```python
from build123d import *

# Parameters (mm, degrees)
SKETCH_2_R          = 19
SKETCH_2_R_2        = 2.75
EXTRUDE_1_DEPTH     = 14
SKETCH_3_R          = 21.125
CUT_EXTRUDE_1_DEPTH = 12.15
FILLET_1_R          = 8
SKETCH_5_R          = 0.9
CUT_EXTRUDE_3_DEPTH = 61.017185039
SKETCH_6_R          = 21.125
SKETCH_6_R_2        = 2.75
EXTRUDE_2_DEPTH     = 14
CUT_EXTRUDE_4_DEPTH = 13
SKETCH_8_R          = 2
CUT_EXTRUDE_5_DEPTH = 2
FILLET_2_R          = 1
CUT_EXTRUDE_6_REACH = 77.034
CHAMFER_1_SIZE      = 1


with BuildPart() as part:
    # Эскиз2 → Бобышка-Вытянуть1 (new body)
    with BuildSketch(Plane.XY):
        with BuildLine():
            ThreePointArc((26, 26.25), (0, 52.25), (-26, 26.25))
            Line((-26, 26.25), (-26, -20))
            Line((-26, -20), (26, -20))
            Line((26, -20), (26, 26.25))
        make_face()
        with Locations((0, 26.25)):
            Circle(SKETCH_2_R, mode=Mode.SUBTRACT)
        with Locations((12, -10)):
            Circle(SKETCH_2_R_2, mode=Mode.SUBTRACT)
        with Locations((-12, -10)):
            Circle(SKETCH_2_R_2, mode=Mode.SUBTRACT)
    extrude(amount=EXTRUDE_1_DEPTH)

    # Эскиз3 → Вырез-Вытянуть1 (cut)
    with BuildSketch(Plane.XY.offset(14)):
        with Locations((0, 26.25)):
            Circle(SKETCH_3_R)
    extrude(amount=-CUT_EXTRUDE_1_DEPTH, mode=Mode.SUBTRACT)

    # Скругление1
    fillet_1_edges = [part.edges().sort_by_distance(p)[0] for p in [
        (26, -20, 7),
        (-26, -20, 7),
    ]]
    fillet(fillet_1_edges, radius=FILLET_1_R)

    # Эскиз5 → Вырез-Вытянуть3 (cut, through all)
    with BuildSketch(Plane.XY.offset(14)):
        with Locations((0, 49.75)):
            Circle(SKETCH_5_R)
        with Locations((-23.5, 26.25)):
            Circle(SKETCH_5_R)
        with Locations((23.5, 26.25)):
            Circle(SKETCH_5_R)
        with Locations((-22, -10)):
            Circle(SKETCH_5_R)
        with Locations(Location((22, -10, 0), (0, 0, 180))):
            Circle(SKETCH_5_R)
    extrude(amount=-CUT_EXTRUDE_3_DEPTH, mode=Mode.SUBTRACT)

    # Эскиз6 → Бобышка-Вытянуть2 (add, through all)
    with BuildSketch(Plane.XY.offset(14)):
        with Locations((0, 26.25)):
            Circle(SKETCH_6_R)
        with Locations((-12, -10)):
            Circle(SKETCH_6_R_2)
        with Locations((12, -10)):
            Circle(SKETCH_6_R_2)
    extrude(amount=-EXTRUDE_2_DEPTH)

    # Эскиз7 → Вырез-Вытянуть4 (cut)
    with BuildSketch(Plane(origin=(0, 0, 0), x_dir=(-1, 0, 0), z_dir=(0, 0, -1))):
        with BuildLine():
            Line((-23.5, 21.75), (-24, 21.75))
            Line((-24, 21.75), (-24, -5.5))
            Line((-24, -5.5), (-22, -5.5))
            ThreePointArc((-22, -5.5), (-18.818019485, -6.818019485), (-17.5, -10))
            Line((-17.5, -10), (-17.5, -18))
            Line((-17.5, -18), (17.5, -18))
            Line((17.5, -18), (17.5, -10))
            ThreePointArc((17.5, -10), (18.818019485, -6.818019485), (22, -5.5))
            Line((22, -5.5), (24, -5.5))
            Line((24, -5.5), (24, 21.75))
            Line((24, 21.75), (23.5, 21.75))
            ThreePointArc((23.5, 21.75), (20.318019485, 23.068019485), (19, 26.25))
            ThreePointArc((19, 26.25), (0, 45.25), (-19, 26.25))
            ThreePointArc((-19, 26.25), (-20.318019485, 23.068019485), (-23.5, 21.75))
        make_face()
    extrude(amount=-CUT_EXTRUDE_4_DEPTH, mode=Mode.SUBTRACT)

    # Эскиз8 → Вырез-Вытянуть5 (cut)
    with BuildSketch(Plane.XY.offset(14)):
        with Locations((-22, -10)):
            Circle(SKETCH_8_R)
        with Locations((22, -10)):
            Circle(SKETCH_8_R)
        with BuildLine():
            Line((2, 49.75), (2, 52.25))
            Line((2, 52.25), (-2, 52.25))
            Line((-2, 52.25), (-2, 49.75))
            ThreePointArc((-2, 49.75), (0, 47.75), (2, 49.75))
        make_face()
        with BuildLine():
            Line((26, 28.25), (23.5, 28.25))
            ThreePointArc((23.5, 28.25), (21.5, 26.25), (23.5, 24.25))
            Line((23.5, 24.25), (26, 24.25))
            Line((26, 24.25), (26, 28.25))
        make_face()
        with BuildLine():
            Line((-26, 24.25), (-23.5, 24.25))
            ThreePointArc((-23.5, 24.25), (-21.5, 26.25), (-23.5, 28.25))
            Line((-23.5, 28.25), (-26, 28.25))
            Line((-26, 28.25), (-26, 24.25))
        make_face()
    extrude(amount=-CUT_EXTRUDE_5_DEPTH, mode=Mode.SUBTRACT)

    # Скругление2
    fillet_2_edges = [part.edges().sort_by_distance(p)[0] for p in [
        (24, -5.5, 6.5),
        (17.5, -18, 6.5),
        (-17.5, -18, 6.5),
        (-24, -5.5, 6.5),
        (-24, 21.75, 6.5),
        (24, 21.75, 6.5),
        (26, 24.25, 13),
        (25.922962794, 28.25, 13),
        (2, 52.172962794, 13),
        (-2, 52.172962794, 13),
        (-26, 24.25, 13),
        (-25.922962794, 28.25, 13),
    ]]
    fillet(fillet_2_edges, radius=FILLET_2_R)

    # Эскиз9 → Вырез-Вытянуть6 (cut, up to next)
    with BuildSketch(Plane.ZY.offset(26), mode=Mode.PRIVATE) as cut_extrude_6_sk1:
        with BuildLine():
            Line((-7.5, 10.375), (4.5, 10.375))
            ThreePointArc((4.5, 10.375), (6.621320344, 9.496320344), (7.5, 7.375))
            Line((7.5, 7.375), (7.5, 6.875))
            ThreePointArc((7.5, 6.875), (6.621320344, 4.753679656), (4.5, 3.875))
            Line((4.5, 3.875), (-7.5, 3.875))
            Line((-7.5, 3.875), (-7.5, 10.375))
        make_face()
    cut_extrude_6_tool1 = extrude(cut_extrude_6_sk1.sketch, amount=-CUT_EXTRUDE_6_REACH, mode=Mode.PRIVATE) & part.part
    add(cut_extrude_6_tool1.solids().sort_by_distance((-26, 7.125, -0.281755))[0], mode=Mode.SUBTRACT)

    # Фаска1
    chamfer_1_edges = [part.edges().sort_by_distance(p)[0] for p in [
        (2, 50.409673646, 14),
        (0, 47.75, 14),
        (21.5, 26.25, 14),
        (24.25, 24.25, 14),
        (-24.159673646, 28.25, 14),
        (-21.5, 26.25, 14),
        (22.5, -5.5, 13),
        (24, 8.136387212, 13),
        (0, -18, 13),
        (-17.5, -13.5, 13),
        (-24, 8.136387212, 13),
        (-20.176529744, 23.216100619, 13),
        (23.738548946, 21.446974287, 13),
        (-23.738548945, 21.446974288, 13),
        (-23.707106781, -5.207106781, 13),
        (-17.207106781, -17.707106781, 13),
        (17.207106781, -17.707106781, 13),
        (23.707106781, -5.207106781, 13),
        (26, 5.625, 14),
        (-2, 50.409673646, 14),
        (-18.384776311, 44.634776311, 14),
        (-24.25, 24.25, 14),
        (-26, 5.625, 14),
        (24.159673646, 28.25, 14),
        (18.384776311, 44.634776311, 14),
        (-25.567678769, 28.586675042, 14),
        (-25.707106781, 23.957106781, 14),
        (-2.336675042, 51.817678769, 14),
        (2.336675042, 51.817678769, 14),
        (25.567678769, 28.586675042, 14),
        (25.707106781, 23.957106781, 14),
        (0, -20, 14),
        (23.656854249, -17.656854249, 14),
        (-23.656854249, -17.656854249, 14),
        (20.176529744, 23.216100619, 13),
        (0, 45.25, 13),
        (-22.5, -5.5, 13),
        (-18.818019485, -6.818019485, 13),
        (17.5, -13.5, 13),
        (18.818019485, -6.818019485, 13),
    ]]
    chamfer(chamfer_1_edges, length=CHAMFER_1_SIZE - 0.0001)  # a hair under: the kernel refuses the full size


solid = part.part
```
Work out the finished part from the listing and answer in its coordinate system (mm). A direction names the side the tool comes from. Give positions to 0.01 mm unless a question says otherwise; leave off trailing zeros. Loops run counter-clockwise (first coordinate to the right, second up) from the corner with the lowest first, then second, coordinate; pieces in that order, holes last. Notation, with made-up numbers: (-11, 43.25) -> (14, 43.25) arc R29 ccw to (14, 64.25) -> close; hole circle Ø6 at (72, 13.25). An arc over 180 degrees is marked (long way). One line per question, with ' | ' between items. Start each with the question number.
1) Section B-B, the plane z = 9.5 is taken. State how many separate pieces and enclosed holes the cut face has, then the cut area to 3 significant figures.
2) For faces 4 (the face through (-0.04, 47.75, 12.51)), 5 (the face through (-25, 3.875, 2)), 6 (the face through (21.5, 26.3, 12.5)), 7 (the face through (0, 14, 13)), 8 (the face through (-23.474, -8.648, 13.014)), determine the directions among +Z, -Z, +X, -X, +Y, -Y from which every point of the face is accessible in a straight line to the end or side of a thin tool.
3) Straight lines are drawn through the part: L1, parallel to Y at x = 0, z = 6.25; L2, parallel to Y at x = 22, z = 13.25; L3, parallel to Y at x = 22, z = 12.95. For each, find the intervals that lie inside material, in ascending order.
4) Each of these flat-tipped pins is pushed along its axis until it touches: pin 1 (6 mm diameter, centred on x = 0, y = 2.5, fed in from -Z); pin 2 (2 mm diameter, centred on x = -22, y = -10, fed in from +Z); pin 3 (8 mm diameter, centred on y = 35, z = 10.5, fed in from -X). Where does it stop, or does it pass through?
5) Section A-A, the plane x = 0 is taken. Determine the outline of the cut face in (y, z).
6) Determine the mould class of faces 1 (the face through (0, -18, 6)), 2 (the face through (0, -20, 6)), 3 (the face through (-23.719, -17.594, 6.591)) for opening direction X: +X half, -X half, draft (parallel to the pull), parting line (faces both ways), or undercut.
Resolved:
1) separate pieces: 1 | enclosed holes: 6 | area: 927 mm2
2) face 4: +Z, +Y | face 5: -Z, -X | face 6: +Z, +X | face 7: -Z | face 8: +Z
3) L1: -20 to -18, 45.25 to 48.85, 50.65 to 52.25 | L2: -18.64 to -12, -8 to 24.57, 27.93 to 39.63 | L3: -18.93 to -12, -8 to -4.55, 21.01 to 24.93, 27.57 to 40.11
4) pin 1: z = 13 | pin 2: z = 12 | pin 3: x = -25.56
5) outline: (-20, 0) -> (-18, 0) -> (-18, 12) -> (-17, 13) -> (44.25, 13) -> (45.25, 12) -> (45.25, 0) -> (48.85, 0) -> (48.85, 12) -> (47.75, 12) -> (47.75, 13) -> (46.75, 14) -> (-19, 14) -> (-20, 13) -> close; (50.65, 0) -> (52.25, 0) -> (52.25, 12) -> (50.65, 12) -> close
6) face 1: undercut | face 2: draft | face 3: -X half
